from build123d import *

# Parameters (mm, degrees)
SKETCH1_W           = 234
SKETCH1_H           = 164
BOSS_EXTRUDE1_DEPTH = 151
SKETCH2_W           = 134.536158908
SKETCH2_H           = 46.032358143
CUT_EXTRUDE1_DEPTH  = 291.311901237
FILLET1_R           = 40
SKETCH3_W           = 18
SKETCH3_H           = 30
BOSS_EXTRUDE2_DEPTH = 70
SKETCH4_R           = 3
CUT_EXTRUDE2_DEPTH  = 214.07510413


with BuildPart() as part:
    # Sketch1 → Boss-Extrude1 (new body)
    with BuildSketch(Plane(origin=(0, 0, 0), x_dir=(1, 0, 0), z_dir=(0, 1, 0))):
        Rectangle(SKETCH1_W, SKETCH1_H)
    extrude(amount=BOSS_EXTRUDE1_DEPTH)

    # Sketch2 → Cut-Extrude1 (cut, through all)
    with BuildSketch(Plane.ZY.offset(117)):
        with Locations((48.268079454, 5.983820929)):
            Rectangle(SKETCH2_W, SKETCH2_H)
    extrude(amount=-CUT_EXTRUDE1_DEPTH, mode=Mode.SUBTRACT)

    # Fillet1
    fillet1_edges = [part.edges().sort_by_distance(p)[0] for p in [
        (-117, 75.5, -82),
        (117, 75.5, -82),
    ]]
    fillet(fillet1_edges, radius=FILLET1_R)

    # Sketch3 → Boss-Extrude2 (add)
    with BuildSketch(Plane.XZ.offset(-29)):
        with Locations((0, -2)):
            Rectangle(SKETCH3_W, SKETCH3_H)
    extrude(amount=BOSS_EXTRUDE2_DEPTH)

    # Sketch4 → Cut-Extrude2 (cut, through all)
    with BuildSketch(Plane.ZY.offset(9)):
        with Locations((0, -31)):
            Circle(SKETCH4_R)
    extrude(amount=-CUT_EXTRUDE2_DEPTH, mode=Mode.SUBTRACT)


solid = part.part
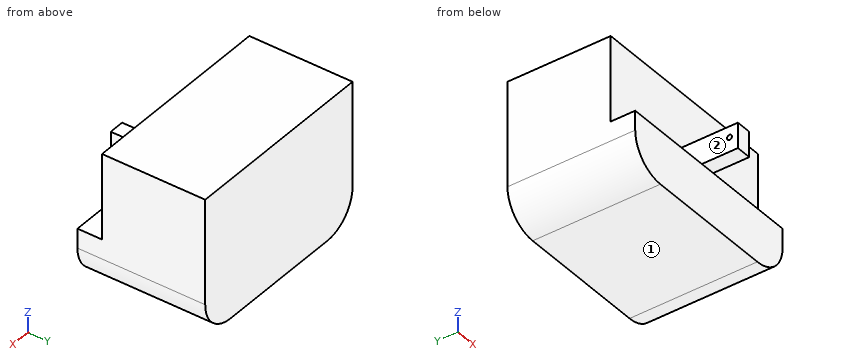
Model file for the job. Use its own axes, mm. Face numbers are marked on the shaded views. A direction names the side the tool comes from. Round coordinates to 2 decimals unless told otherwise and drop trailing zeros. Loops run counter-clockwise (first coordinate to the right, second up) from the corner with the lowest first, then second, coordinate; pieces in that order, holes last. Notation, with made-up numbers: (52.25, 57) -> (87.25, 57) arc R23 cw to (87.25, 93) -> close; hole circle Ø11 at (28.25, 67.5). An arc over 180 degrees is marked (long way). Answer as CSV lines item,"result". Start each with the question number.
1) Slice it at C-C (x = -3). List the corners of the cut face in (y, z).
2) Tool access for the marked faces 1 and 2: list every direction of +Z, -Z, +X, -X, +Y, -Y with a clear straight run to the whole face (end or side of a thin tool).
3) Slice it at D-D (x = -101). List the corners of the cut face in (y, z).
4) Pin check, flat tips, straight feed: P1, Ø19, axis at x = 20.5, z = -39, coming from the -Y side; P2, Ø15, axis at y = 8.5, z = -8.5, coming from the +X side; P3, Ø6, axis at x = 4.5, y = 14.5, coming from the +Z side. Stop position of each tip, or through.
5) Slice it at A-A (y = -31). List the corners of the cut face in (x, z), plus the area to 3 significant figures.
6) Slice it at B-B (z = 0). List the corners of the cut face in (x, y), plus the area to 3 significant figures.
7) Probe line 1 along Y through (x, z) = (2, 0); line 2 along Z through (x, y) = (-8.5, 4); line 3 along Y through (x, z) = (-14, -28). List the from-to ranges inside material, lowest first.
Filled in:
1,outline,"(-41, -17) -> (29, -17) -> (29, -19) -> (0, -19) -> (0, -82) -> (151, -82) -> (151, 82) -> (29, 82) -> (29, 13) -> (-41, 13) -> close; hole circle Ø6 at (-31, 0)"
2,face 1,"-Z, +X, -X, +Y, -Y"
2,face 2,"+Z, -X, -Y"
3,outline,"(0, -74) -> (151, -74) -> (151, 82) -> (29, 82) -> (29, -19) -> (0, -19) -> close"
4,P1,"stops at y = 0"
4,P2,"stops at x = 9"
4,P3,"stops at z = 13"
5,outline,"(-9, -17) -> (9, -17) -> (9, -3) -> (-9, -3) -> close; (-9, 3) -> (9, 3) -> (9, 13) -> (-9, 13) -> close"
5,area,"432 mm2"
6,outline,"(-117, 29) -> (-9, 29) -> (-9, -28) -> (9, -28) -> (9, 29) -> (117, 29) -> (117, 151) -> (-117, 151) -> close; (-9, -41) -> (9, -41) -> (9, -34) -> (-9, -34) -> close"
6,area,"29,700 mm2"
7,line 1,"y = -41 to -34, -28 to 151"
7,line 2,"z = -82 to -19, -17 to 13"
7,line 3,"y = 0 to 151"
